CAD build for the part. Positions are in the model's coordinates, mm. Round coordinates to 2 decimals unless told otherwise and drop trailing zeros. Loops run counter-clockwise (first coordinate to the right, second up) from the corner with the lowest first, then second, coordinate; pieces in that order, holes last.
from build123d import *

# Parameters (mm, degrees)
F0_W     = 100
F0_H     = 40
F1_DEPTH = 10
F3_DEPTH = 3
F4_R     = 4
F4_R_2   = 3
F5_DEPTH = 10
F6_R     = 5


with BuildPart() as f1:
    # F0 (on Top) → F1 (new body)
    with BuildSketch(Plane.XY):
        Rectangle(F0_W, F0_H)
    extrude(amount=F1_DEPTH)

    # F2 (on face) → F3 (join)
    with BuildSketch(Plane.XY.offset(10)):
        with BuildLine():
            add(Edge.make_bspline(
                [(-35, 4), (-43.660254, 4), (-39.330127, -11), (-35, -26), (-30.669873, -11), (-26.339746, 4), (-35, 4)],
                knots=[0, 0, 0, 2.094395, 2.094395, 4.18879, 4.18879, 6.283185, 6.283185, 6.283185], degree=2, weights=[1, 0.5, 1, 0.5, 1, 0.5, 1]))
        make_face()
        with BuildLine():
            add(Edge.make_bspline(
                [(-8.672845, 7.551938), (-11.516397, 4.286327), (2.914646, -5.408774), (17.345689, -15.103876), (5.758198, -2.143164), (-5.829292, 10.817548), (-8.672845, 7.551938)],
                knots=[0, 0, 0, 2.094395, 2.094395, 4.18879, 4.18879, 6.283185, 6.283185, 6.283185], degree=2, weights=[1, 0.5, 1, 0.5, 1, 0.5, 1]))
        make_face()
    extrude(amount=F3_DEPTH)

    # F4 (on face) → F5 (cut)
    with BuildSketch(Plane.XY.offset(10)):
        with Locations((40, 10)):
            Circle(F4_R)
        with Locations((42, -12)):
            Circle(F4_R_2)
    extrude(amount=-F5_DEPTH, mode=Mode.SUBTRACT)

    # F6
    f6_edges = [f1.edges().sort_by_distance(p)[0] for p in [
        (-50, -20, 5),
        (-50, 20, 5),
        (50, 20, 5),
        (50, -20, 5),
    ]]
    fillet(f6_edges, radius=F6_R)


solid = f1.part
Item 1: Cut at B-B (z = 3.5). List the corners of the cut face in (x, y).
Verdict:
outline: (-50, -15) arc R5 ccw to (-45, -20) - (45, -20) arc R5 ccw to (50, -15) - (50, 15) arc R5 ccw to (45, 20) - (-45, 20) arc R5 ccw to (-50, 15) - close; hole circle Ø8 at (40, 10); hole circle Ø6 at (42, -12)
Item 2: Cut at C-C (x = 42). List the corners of the cut face in (y, z), plus the area to 3 significant figures.
Verdict:
outline: (-20, 0) - (-15, 0) - (-15, 10) - (-20, 10) - close; (-9, 0) - (6.54, 0) - (6.54, 10) - (-9, 10) - close; (13.46, 0) - (20, 0) - (20, 10) - (13.46, 10) - close
area: 271 mm2
Item 3: Cut at D-D (x = 29). List the corners of the cut face in (y, z).
Verdict:
outline: (-20, 0) - (20, 0) - (20, 10) - (-20, 10) - close
Item 4: Wall check: L1, parallel to Y at x = 40, z = 6.5; L2, parallel to Z at x = -7, y = 3.5; L3, parallel to X at y = 12, z = 3. Give the ranges that are in metal, low to high.
Verdict:
L1: y = -20 to -14.24, -9.76 to 6, 14 to 20
L2: z = 0 to 10
L3: x = -50 to 36.54, 43.46 to 50
Item 5: Flat gauge pin, fed straight in: P1, Ø7, axis at x = 40, y = 10, coming from the +Z side. Where does the tip first touch, or does it go through?
Verdict:
P1: passes through
Item 6: Mould opens along X. For faces 1 (the cylindrical face through (39, -12, 5)), 2 (the flat face through (-1, 0, 0)), 3 (the cylindrical face through (36, 10, 5)), 4 (the cylindrical face through (-49, 18, 5)) say: released by +X, released by -X, zero draft, split by the parting line, or undercut.
Verdict:
face 1: undercut
face 2: zero draft
face 3: undercut
face 4: released by -X
Item 7: Cut at A-A (y = 10). List the corners of the cut face in (x, z), plus the area to 3 significant figures.
Verdict:
outline: (-50, 0) - (36, 0) - (36, 10) - (-50, 10) - close; (44, 0) - (50, 0) - (50, 10) - (44, 10) - close
area: 920 mm2
